```python
from build123d import *

# Parameters (mm, degrees)
SKETCH1_R           = 11.55
SKETCH1_R_2         = 8.55
BOSS_EXTRUDE1_DEPTH = 12
BOSS_EXTRUDE2_DEPTH = 4
SKETCH3_R           = 11.55
SKETCH3_R_2         = 8.55
BOSS_EXTRUDE3_DEPTH = 4
SKETCH4_R           = 11.55
SKETCH4_R_2         = 8.55
BOSS_EXTRUDE4_DEPTH = 20


with BuildPart() as part:
    # Sketch1 → Boss-Extrude1 (new body)
    with BuildSketch(Plane(origin=(0, 0, 0), x_dir=(0, 0, -1), z_dir=(1, 0, 0))):
        Circle(SKETCH1_R)
        Circle(SKETCH1_R_2, mode=Mode.SUBTRACT)
    extrude(amount=BOSS_EXTRUDE1_DEPTH)



with BuildPart() as body_2:
    # Sketch2 → Boss-Extrude2 (new body)
    with BuildSketch(Plane(origin=(12, 0, 0), x_dir=(0, 0, -1), z_dir=(1, 0, 0))):
        with BuildLine():
            Line((-3.65, 7.731752712), (-3.65, -7.731752712))
            ThreePointArc((-3.65, -7.731752712), (0, -8.55), (3.65, -7.731752712))
            Line((3.65, -7.731752712), (3.65, 7.731752712))
            ThreePointArc((3.65, 7.731752712), (0, 8.55), (-3.65, 7.731752712))
        make_face()
    extrude(amount=BOSS_EXTRUDE2_DEPTH)


with BuildPart() as part_1:
    add(part.part)

    add(body_2.part)  # Boss-Extrude3 merges body 2
    # Sketch3 → Boss-Extrude3 (add)
    with BuildSketch(Plane(origin=(12, 0, 0), x_dir=(0, 0, -1), z_dir=(1, 0, 0))):
        Circle(SKETCH3_R)
        with Locations(Location((0, 0, 0), (0, 0, 244.72897634))):
            Circle(SKETCH3_R_2, mode=Mode.SUBTRACT)
    extrude(amount=BOSS_EXTRUDE3_DEPTH)

    # Sketch4 → Boss-Extrude4 (add)
    with BuildSketch(Plane(origin=(16, 0, 0), x_dir=(0, 0, -1), z_dir=(1, 0, 0))):
        Circle(SKETCH4_R)
        Circle(SKETCH4_R_2, mode=Mode.SUBTRACT)
    extrude(amount=BOSS_EXTRUDE4_DEPTH)


solid = part_1.part
```
For this review, take the finished solid that the model builds, in its own axes (mm). A direction names the side the tool comes from. Round coordinates to 2 decimals unless told otherwise and drop trailing zeros. Write each loop counter-clockwise with the first axis right and the second up, starting at its lowest first coordinate (ties: lowest second). Pieces come first, ordered by that corner, then holes. Notation, with made-up numbers: (54, 34.25) - (68, 34.25) arc R9 cw to (68, 45.25) - close; hole circle Ø5 at (-16, 35.5). An arc over 180 degrees is marked (long way). Answer as a JSON object with one key per item and string values.
1. We need section C-C on x = 21.5. Give the boundary of the cut face in (y, z), then the cut area to 3 significant figures.
Response values:
{"outline": "circle Ø23.1 at (0, 0); hole circle Ø17.1 at (0, 0)", "area": "189 mm2"}
2. Tool access review of faces 1 (the face through (12, 0, 0)), 2 (the face through (0, 0, 9)), 3 (the face through (14, 0, 3.65)): name each direction out of +Z, -Z, +X, -X, +Y, -Y from which nothing blocks a thin tool from reaching the whole face with its end or side.
Response values:
{"face 1": "-X", "face 2": "+Z, -Z, -X, +Y, -Y", "face 3": "+X, -X"}
3. We need section D-D on y = 5.75. Give the boundary of the cut face in (x, z), then the cut area to 3 significant figures.
Response values:
{"outline": "(0, -10.02) - (36, -10.02) - (36, -6.33) - (0, -6.33) - close; (0, 6.33) - (36, 6.33) - (36, 10.02) - (0, 10.02) - close; (12, -3.65) - (16, -3.65) - (16, 3.65) - (12, 3.65) - close", "area": "295 mm2"}
4. We need section B-B on z = 0. Give the boundary of the cut face in (x, y), then the cut area to 3 significant figures.
Response values:
{"outline": "(0, -11.55) - (36, -11.55) - (36, -8.55) - (16, -8.55) - (16, 8.55) - (36, 8.55) - (36, 11.55) - (0, 11.55) - (0, 8.55) - (12, 8.55) - (12, -8.55) - (0, -8.55) - close", "area": "284 mm2"}
5. For pin 1 Ø6 at (y, z) = (-3.5, -1.5) entering from +X; pin 2 Ø1 at (x, z) = (4, 4) entering from -Y; pin 3 Ø1.2 at (x, y) = (13, -3.5) entering from -Z, all flat-tipped, find the tip position at first contact; note any pin that passes through.
Response values:
{"pin 1": "stops at x = 16", "pin 2": "stops at y = -11.01", "pin 3": "stops at z = -11.18"}
6. Draft analysis for pull direction Y (two halves, no side actions). For faces 4 (the face through (17.748, -11.275, 2.504)), 5 (the face through (14, 0, -3.65)), 6 (the face through (36, 0, 9)), state which applies: +Y half, -Y half, draft (parallel to the pull), parting line (faces both ways), or undercut.
Response values:
{"face 4": "parting line", "face 5": "undercut", "face 6": "draft"}
7. To check wall thickness, follow line 1 along Y through (x, z) = (18.5, 0); line 2 along Z through (x, y) = (8, -3.5); line 3 along Z through (x, y) = (27, 5). State the ranges of each line that lie inside material, in increasing order.
Response values:
{"line 1": "y = -11.55 to -8.55, 8.55 to 11.55", "line 2": "z = -11.01 to -7.8, 7.8 to 11.01", "line 3": "z = -10.41 to -6.94, 6.94 to 10.41"}
